Verification items for the finished model (mm, model axes). Face numbers are marked on the shaded views. A direction names the side the tool comes from. Give positions to 0.01 mm unless a question says otherwise; leave off trailing zeros. Write each loop counter-clockwise with the first axis right and the second up, starting at its lowest first coordinate (ties: lowest second). Pieces come first, ordered by that corner, then holes. Notation, with made-up numbers: (0.5, -14) -> (24.5, -14) arc R20 ccw to (24.5, 19) -> close; hole circle Ø11 at (-16.5, -11). An arc over 180 degrees is marked (long way). Answer as CSV lines item,"result". Start each with the question number.
1) Sectioned sample at A-A on y = 3. Record the cut outline in (x, z).
2) Sectioned sample at B-B on x = -20.3. Record the cut outline in (y, z), and give its area (3 significant figures).
3) Sectioned sample at D-D on z = -25. Record the cut outline in (x, y), and give its area (3 significant figures).
4) Gauge pin test, flat ends, axial feed: pin 1 Ø1.8 at (x, y) = (25.5, 3) entering from -Z; pin 2 Ø0.7 at (y, z) = (0.5, -14) entering from +X; pin 3 Ø5 at (x, z) = (-23.5, 18) entering from +Y. Record the tip position at first contact, or that the pin passes through.
5) Tool access check on the marked faces 1 and 2. Record the directions out of +Z, -Z, +X, -X, +Y, -Y that give a thin tool (end or side, any length) a straight path to the whole face; none if there is none.
6) Material ranges on L1, parallel to X at y = 0.45, z = -29; L2, parallel to Y at x = 31, z = 14; L3, parallel to X at y = 6, z = 1, recorded low to high.
7) Sectioned sample at C-C on z = 20. Record the cut outline in (x, y), and give its area (3 significant figures).
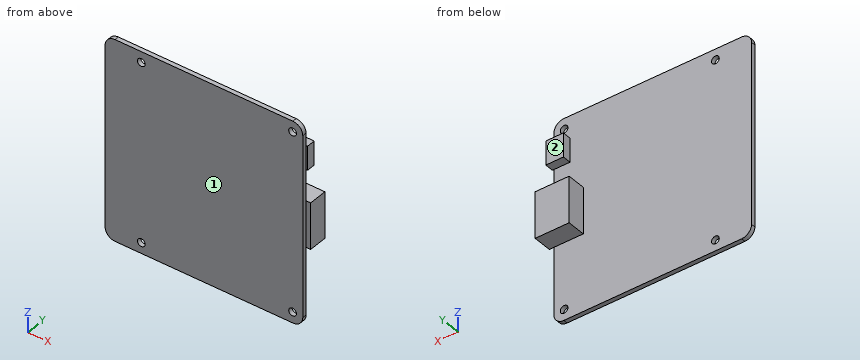
```python
from build123d import *

# Parameters (mm, degrees)
SKETCH1_W           = 64
SKETCH1_H           = 65
SKETCH1_R           = 1.25
BOSS_EXTRUDE1_DEPTH = 1.4
SKETCH2_W           = 11
SKETCH2_H           = 15
BOSS_EXTRUDE2_DEPTH = 6
SKETCH3_W           = 5.7
SKETCH3_H           = 7.75
BOSS_EXTRUDE3_DEPTH = 2.8
FILLET1_R           = 3.2


with BuildPart() as part:
    # Sketch1 → Boss-Extrude1 (new body)
    with BuildSketch(Plane(origin=(0, 0, 0), x_dir=(1, 0, 0), z_dir=(0, 1, 0))):
        Rectangle(SKETCH1_W, SKETCH1_H)
        with Locations(Location((28.7, -29, 0), (0, 0, 270))):
            Circle(SKETCH1_R, mode=Mode.SUBTRACT)
        with Locations(Location((-20.3, -29, 0), (0, 0, 270))):
            Circle(SKETCH1_R, mode=Mode.SUBTRACT)
        with Locations(Location((-20.3, 29, 0), (0, 0, 270))):
            Circle(SKETCH1_R, mode=Mode.SUBTRACT)
        with Locations(Location((28.7, 29, 0), (0, 0, 270))):
            Circle(SKETCH1_R, mode=Mode.SUBTRACT)
    extrude(amount=BOSS_EXTRUDE1_DEPTH)

    # Sketch2 → Boss-Extrude2 (add)
    with BuildSketch(Plane(origin=(0, 1.4, 0), x_dir=(1, 0, 0), z_dir=(0, 1, 0))):
        with Locations((28, 0)):
            Rectangle(SKETCH2_W, SKETCH2_H)
    extrude(amount=BOSS_EXTRUDE2_DEPTH)

    # Sketch3 → Boss-Extrude3 (add)
    with BuildSketch(Plane(origin=(0, 1.4, 0), x_dir=(1, 0, 0), z_dir=(0, 1, 0))):
        with Locations((29.65, -21.425)):
            Rectangle(SKETCH3_W, SKETCH3_H)
    extrude(amount=BOSS_EXTRUDE3_DEPTH)

    # Fillet1
    fillet1_edges = [part.edges().sort_by_distance(p)[0] for p in [
        (32, 0.7, 32.5),
        (-32, 0.7, 32.5),
        (-32, 0.7, -32.5),
        (32, 0.7, -32.5),
    ]]
    fillet(fillet1_edges, radius=FILLET1_R)


solid = part.part
```
Ans:
1,outline,"(22.5, -7.5) -> (33.5, -7.5) -> (33.5, 7.5) -> (22.5, 7.5) -> close; (26.8, 17.55) -> (32.5, 17.55) -> (32.5, 25.3) -> (26.8, 25.3) -> close"
2,outline,"(0, -32.5) -> (1.4, -32.5) -> (1.4, -30.25) -> (0, -30.25) -> close; (0, -27.75) -> (1.4, -27.75) -> (1.4, 27.75) -> (0, 27.75) -> close; (0, 30.25) -> (1.4, 30.25) -> (1.4, 32.5) -> (0, 32.5) -> close"
2,area,"84.0 mm²"
3,outline,"(-32, 0) -> (32, 0) -> (32, 1.4) -> (-32, 1.4) -> close"
3,area,"89.6 mm²"
4,pin 1,"stops at z = -7.5"
4,pin 2,"stops at x = 32"
4,pin 3,"stops at y = 1.4"
5,face 1,"+Z, -Z, +X, -X, -Y"
5,face 2,"+Z, +X, -X, +Y"
6,L1,"x = -32 to -21.55, -19.05 to 27.45, 29.95 to 32"
6,L2,"y = 0 to 1.4"
6,L3,"x = 22.5 to 33.5"
7,outline,"(-32, 0) -> (32, 0) -> (32, 1.4) -> (32.5, 1.4) -> (32.5, 4.2) -> (26.8, 4.2) -> (26.8, 1.4) -> (-32, 1.4) -> close"
7,area,"106 mm²"
